Check sheet for the modelled part. Datum: model origin and axes. Units: mm. A direction names the side the tool comes from. Round coordinates to 2 decimals unless told otherwise and drop trailing zeros. Loops run counter-clockwise (first coordinate to the right, second up) from the corner with the lowest first, then second, coordinate; pieces in that order, holes last. Notation, with made-up numbers: M -8,-28 L 2,-28 A28 ccw 2,5 Z; hole C 27.25,53 d8. An arc over 180 degrees is marked long. Write item = value, one per line. Start each with the question number.
(1) Cross-section at A-A on z = 0. Record the boundary of the cut face in (x, y).
(2) Scan lines: L1, parallel to X at y = 30.5, z = 0; L2, parallel to X at y = 3.5, z = 0; L3, parallel to Y at x = 23, z = -21.5. Record each from-to range of solid material in increasing order. Write a range as from..to.
(3) Set-up check for faces 5 (the face through (31, 70, -11)), 6 (the face through (9.76, 40.42, 31)): record each of +Z, -Z, +X, -X, +Y, -Y from which the full face is reachable in a straight line by a thin tool's end or side.
(4) Mould release check, pull along X, two halves, no side actions. Record for faces 1 (the face through (-16, 0, -1)), 2 (the face through (-5.554, 4.93, -13.394)), 3 (the face through (-22.818, 34.51, -29.759)), 4 (the face through (-7, 10, 14)): pulls with the +X half, pulls with the -X half, needs draft (parallel to the pull), parting line crosses it, or undercut.
(5) Go/stop test with flat-tipped pins: P1, Ø2, axis at x = 6.5, y = 39, coming from the -Z side; P2, Ø19.5, axis at x = 2.5, z = -12.5, coming from the +Y side; P3, Ø12, axis at y = 44, z = -3.5, coming from the -X side. Record where each tip stops, or that it passes through.
(6) Cross-section at C-C on y = 18.5. Record the boundary of the cut face in (x, z).
(7) Cross-section at D-D on x = 24. Record the boundary of the cut face in (y, z), plus the area to 3 significant figures.
(8) Cross-section at B-B on x = 0. Record the boundary of the cut face in (y, z).
from build123d import *

# Parameters (mm, degrees)
SKETCH_1_R          = 37.5
EXTRUDE_1_DEPTH     = 70
SKETCH_2_R          = 32.5
CUT_EXTRUDE_1_DEPTH = 60
SKETCH_3_R          = 14.5
CUT_EXTRUDE_2_DEPTH = 40


with BuildPart() as part:
    # 草图1 → 凸台-拉伸1 (new body)
    with BuildSketch(Plane(origin=(0, 0, 0), x_dir=(1, 0, 0), z_dir=(0, 1, 0))):
        with Locations(Location((0, 0, 0), (0, 0, 270))):
            Circle(SKETCH_1_R)
    extrude(amount=EXTRUDE_1_DEPTH)

    # 草图2 → 切除-拉伸1 (cut)
    with BuildSketch(Plane(origin=(0, 70, 0), x_dir=(1, 0, 0), z_dir=(0, 1, 0))):
        with Locations(Location((0, 0, 0), (0, 0, 270))):
            Circle(SKETCH_2_R)
    extrude(amount=-CUT_EXTRUDE_1_DEPTH, mode=Mode.SUBTRACT)

    # 草图3 → 切除-拉伸2 (cut)
    with BuildSketch(Plane.XZ):
        with Locations(Location((0, 0, 0), (0, 0, 270))):
            Circle(SKETCH_3_R)
    extrude(amount=-CUT_EXTRUDE_2_DEPTH, mode=Mode.SUBTRACT)


solid = part.part
Result:
q1.outline = M -37.5,0 L -14.5,0 L -14.5,10 L -32.5,10 L -32.5,70 L -37.5,70 Z; M 14.5,0 L 37.5,0 L 37.5,70 L 32.5,70 L 32.5,10 L 14.5,10 Z
q2.L1 = -37.5..-32.5, 32.5..37.5
q2.L2 = -37.5..-14.5, 14.5..37.5
q2.L3 = 0..10
q3.face_5 = +Z, -Z, +X, -X, +Y
q3.face_6 = +Y
q4.face_1 = needs draft
q4.face_2 = undercut
q4.face_3 = parting line crosses it
q4.face_4 = undercut
q5.P1 = -37.09
q5.P2 = 10
q5.P3 = -37.5
q6.outline = C 0,0 d75; hole C 0,0 d65
q7.outline = M 0,-28.81 L 70,-28.81 L 70,-21.91 L 10,-21.91 L 10,21.91 L 70,21.91 L 70,28.81 L 0,28.81 Z
q7.area = 1,400 mm^2
q8.outline = M 0,-37.5 L 70,-37.5 L 70,-32.5 L 10,-32.5 L 10,-14.5 L 0,-14.5 Z; M 0,14.5 L 10,14.5 L 10,32.5 L 70,32.5 L 70,37.5 L 0,37.5 Z
